The figure shows three views and two pictorial views of one solid part (mm, origin at its lowest corner). Answer the questions. Coordinates: 2 decimals unless noted, no trailing zeros. Write each loop counter-clockwise with the first axis right and the second up, starting at its lowest first coordinate (ties: lowest second). Pieces come first, ordered by that corner, then holes. Notation, with made-up numbers: (19.25, 77) - (73.25, 77) arc R26 cw to (73.25, 95) - close; hole circle Ø3 at (76.25, 20.25). An arc over 180 degrees is marked (long way). Use a Markdown table: item, result. Add a question column.
(1) Find the intervals of material crossed by line 1 (X direction, y = 10, z = 1.15); line 2 (Y direction, x = 38, z = 2.65); line 3 (X direction, y = 9, z = 3.75) (1 decimal), in increasing order. Write a range as from..to.
(2) Given pin 1 Ø1.5 at (x, z) = (38, 4) entering from -Y, flat-ended and moving along its own axis, determine where the tip first touches the part or whether it passes through.
(3) The part is cut by section A-A, the plane x = 108. Give the vertices of the cut face in (y, z).
(4) The part is cut by section B-B, the plane y = 10. Give the vertices of the cut face in (x, z).
(5) The part is cut by section C-C, the plane z = 1.4. Give the vertices of the cut face in (x, y), then the cut area to 3 significant figures.
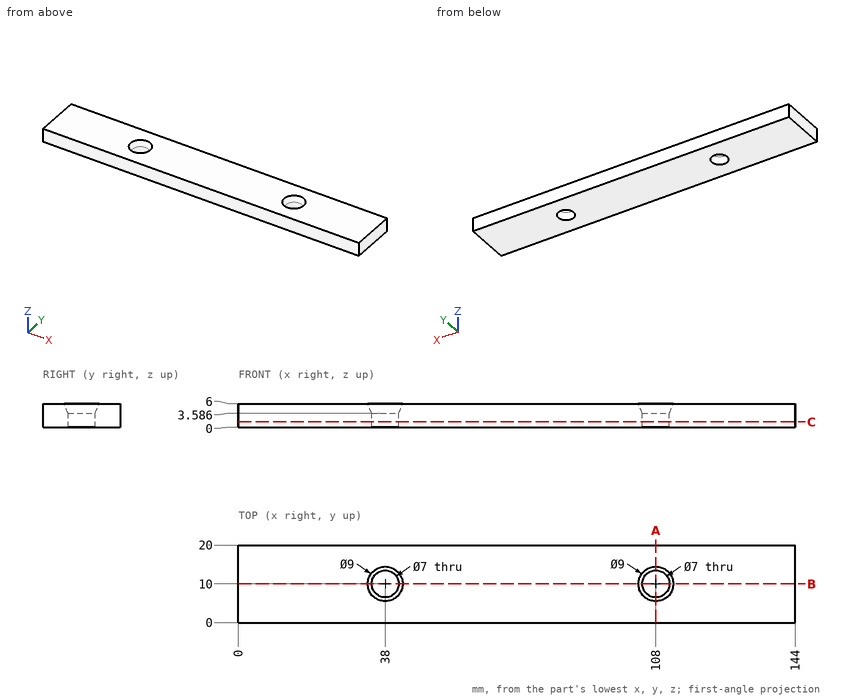
Model answer:
| question | item | result |
|---|---|---|
| 1 | line 1 | 0..34.5, 41.5..104.5, 111.5..144 |
| 1 | line 2 | 0..6.5, 13.5..20 |
| 1 | line 3 | 0..34.6, 41.4..104.6, 111.4..144 |
| 2 | pin 1 | y = 0 |
| 3 | outline | (0, 0) - (6.5, 0) - (6.5, 3.59) - (5.5, 6) - (0, 6) - close; (13.5, 0) - (20, 0) - (20, 6) - (14.5, 6) - (13.5, 3.59) - close |
| 4 | outline | (0, 0) - (34.5, 0) - (34.5, 3.59) - (33.5, 6) - (0, 6) - close; (41.5, 0) - (104.5, 0) - (104.5, 3.59) - (103.5, 6) - (42.5, 6) - (41.5, 3.59) - close; (111.5, 0) - (144, 0) - (144, 6) - (112.5, 6) - (111.5, 3.59) - close |
| 5 | outline | (0, 0) - (144, 0) - (144, 20) - (0, 20) - close; hole circle Ø7 at (38, 10); hole circle Ø7 at (108, 10) |
| 5 | area | 2,800 mm^2 |
